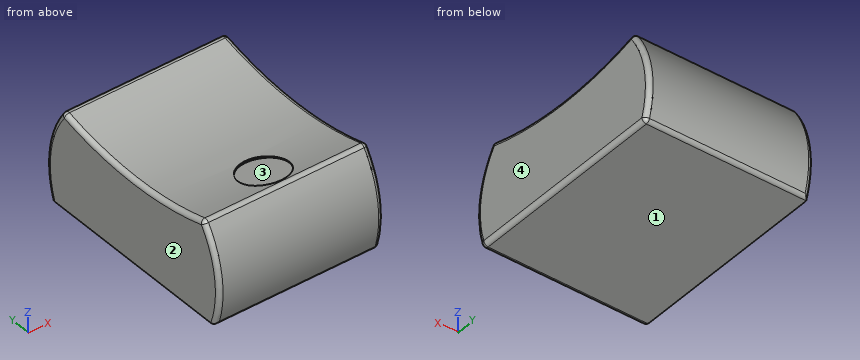
from build123d import *

# Parameters (mm, degrees)
BOSS_EXTRUDE2_DEPTH     = 9.5
FILLET1_R               = 0.5
SKETCH3_R               = 2.71
CUT_EXTRUDE1_DEPTH      = 5.448751278
CUT_EXTRUDE1_DEPTH_BACK = 0.1


with BuildPart() as part:
    # Sketch2 → Boss-Extrude2 (new body, symmetric)
    with BuildSketch(Plane(origin=(0, 0, 0), x_dir=(0, 0, -1), z_dir=(1, 0, 0))):
        with BuildLine():
            Line((0, 12), (0, -12))
            ThreePointArc((0, -12), (-5.710285596, -12.497714363), (-11, -10.29))
            ThreePointArc((-11, -10.29), (-9.540341867, 0), (-11, 10.29))
            ThreePointArc((-11, 10.29), (-5.710285596, 12.497714363), (0, 12))
        make_face()
    extrude(amount=BOSS_EXTRUDE2_DEPTH, both=True)

    # Fillet1
    fillet1_edges = [part.edges().sort_by_distance(p)[0] for p in [
        (9.5, 12.497714363, 5.710285596),
        (9.5, 0, 9.540341867),
        (9.5, -12.497714363, 5.710285596),
        (-9.5, 0, 9.540341867),
        (-9.5, 12.497714363, 5.710285596),
        (-9.5, -12.497714363, 5.710285596),
        (0, -10.29, 11),
        (0, 10.29, 11),
        (0, 12, 0),
        (0, -12, 0),
        (9.5, 0, 0),
    ]]
    fillet(fillet1_edges, radius=FILLET1_R)

    # Sketch3 → Cut-Extrude1 (cut, two sides)
    with BuildSketch(Plane(origin=(0, 1.657226633, 8.525691928), x_dir=(-1, 0, 0), z_dir=(0, 0.190808995, 0.981627183))) as cut_extrude1_sk:
        with Locations((0, 8.947950155)):
            Circle(SKETCH3_R)
    extrude(amount=CUT_EXTRUDE1_DEPTH, mode=Mode.SUBTRACT)
    extrude(cut_extrude1_sk.sketch, amount=-CUT_EXTRUDE1_DEPTH_BACK, mode=Mode.SUBTRACT)


solid = part.part
For this review, take the finished solid that the model builds, in its own axes (mm). Face numbers are marked on the shaded views. Round coordinates to 2 decimals unless told otherwise and drop trailing zeros. Write item = value, one per line. Start each with the question number.
1. Draft analysis for pull direction X (two halves, no side actions). For the marked faces 1, 2, 3 and 4, state which applies: released by +X, released by -X, zero draft, split by the parting line, or undercut.
2. For pin 1 Ø4 at (x, y) = (-6.5, 3.5) entering from +Z; pin 2 Ø3 at (x, z) = (0, 6) entering from -Y; pin 3 Ø4 at (x, z) = (2, 9) entering from -Y, all flat-tipped, find the tip position at first contact; note any pin that passes through.
3. Wall thickness on L1, parallel to Z at x = -1.75, y = 9; L2, parallel to Z at x = 0, y = -0.5; L3, parallel to Y at x = -0.5, z = 4.5: over which ranges is each line inside the solid? List them lowest first.
Evaluation:
q1.face_1 = zero draft
q1.face_2 = released by -X
q1.face_3 = undercut
q1.face_4 = released by +X
q2.pin_1 = 9.95
q2.pin_2 = -12.62
q2.pin_3 = -12.22
q3.L1 = 0 to 10.65
q3.L2 = 0 to 9.54
q3.L3 = -12.62 to 12.62
